Could you check a few things on this drawing? It's one solid part, dimensions in mm from its lowest x, y, z. A direction names the side the tool comes from. Round coordinates to 2 decimals unless told otherwise and drop trailing zeros. Loops run counter-clockwise (first coordinate to the right, second up) from the corner with the lowest first, then second, coordinate; pieces in that order, holes last. Notation, with made-up numbers: M 40.5,-1.75 L 73.5,-1.75 A13 cw 73.5,23.25 Z; hole C 69.5,-10.75 d3. An arc over 180 degrees is marked long. Return JSON: item names as keys, results as strings.
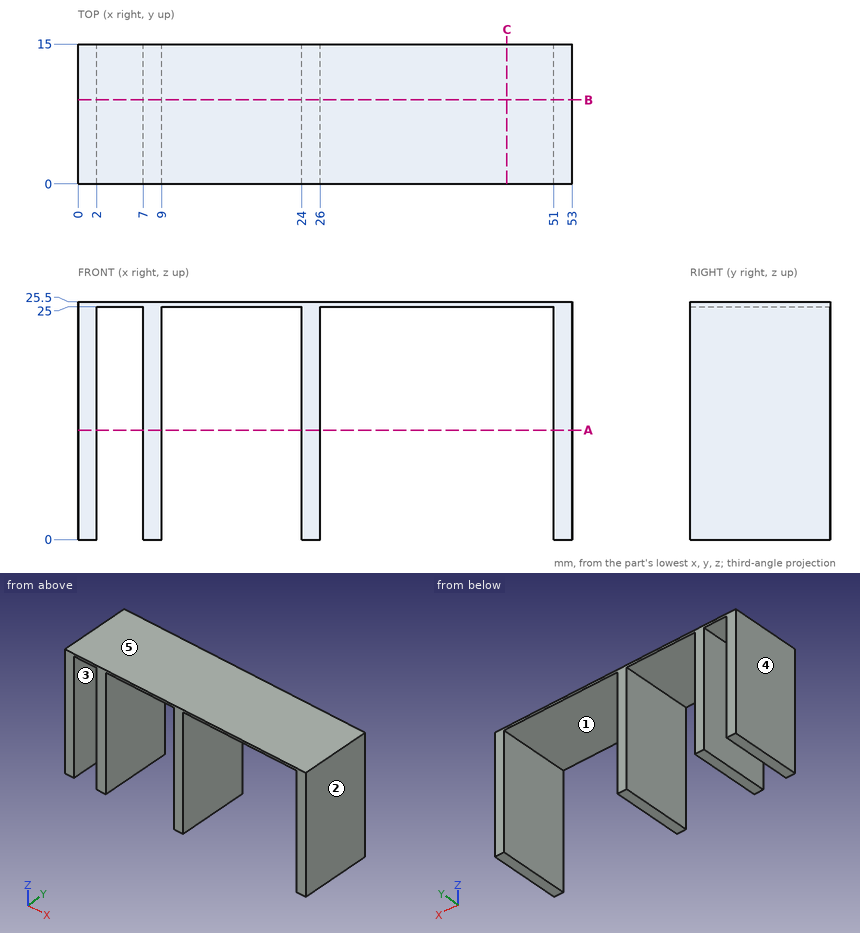
Q1. Suppose I cut it at B-B, the plane y = 9. Please give me the cut outline in (x, z).
Results:
{"outline": "M 0,0 L 2,0 L 2,25 L 7,25 L 7,0 L 9,0 L 9,25 L 24,25 L 24,0 L 26,0 L 26,25 L 51,25 L 51,0 L 53,0 L 53,25.5 L 0,25.5 Z"}
Q2. Thinking about a two-plate mould opening in X: for the marked faces 3, 4 and 5, which applies, pulls with the +X half, pulls with the -X half, needs draft (parallel to the pull), parting line crosses it, or undercut?
Results:
{"face 3": "undercut", "face 4": "pulls with the -X half", "face 5": "needs draft"}
Q3. If I drill on line 1 along X through (y, z) = (4, 12.25); line 2 along Z through (x, y) = (42, 6.5), over which ranges is the centre line in solid material (lowest first)?
Results:
{"line 1": "x = 0 to 2, 7 to 9, 24 to 26, 51 to 53", "line 2": "z = 25 to 25.5"}
Q4. Suppose I cut it at C-C, the plane x = 46. Please give me the cut outline in (y, z), plus the area to 3 significant figures.
Results:
{"outline": "M 0,25 L 15,25 L 15,25.5 L 0,25.5 Z", "area": "7.50 mm2"}
Q5. On a 3-axis mill with a long thin cutter (end or side, diameter ignored), from which of +Z, -Z, +X, -X, +Y, -Y can I reach the whole of each face in a straight line? I mean the marked faces 1 and 2. Say none if no direction works.
Results:
{"face 1": "-Z, +Y, -Y", "face 2": "+Z, -Z, +X, +Y, -Y"}
Q6. I'm going to push a flat-ended pin straight in: pin 1 Ø1 at (x, y) = (29.5, 12.5) entering from -Z. Where does the tip first touch, or does it pass through?
Results:
{"pin 1": "stops at z = 25"}
Q7. Suppose I cut it at A-A, the plane z = 11.75. Please give me the cut outline in (x, y).
Results:
{"outline": "M 0,0 L 2,0 L 2,15 L 0,15 Z; M 7,0 L 9,0 L 9,15 L 7,15 Z; M 24,0 L 26,0 L 26,15 L 24,15 Z; M 51,0 L 53,0 L 53,15 L 51,15 Z"}
